```python
from build123d import *

# Parameters (mm, degrees)
SKETCH1_R           = 3.429
BOSS_EXTRUDE1_DEPTH = 50.8
SKETCH2_W           = 50.8
SKETCH2_H           = 43.18
CUT_EXTRUDE1_DEPTH  = 120.811560377
SKETCH3_R           = 2
CUT_EXTRUDE2_DEPTH  = 114.592253257
FILLET1_START       = -1
FILLET1_DEPTH       = 41.6399999
FILLET1_START_2     = 4.794504
FILLET1_2_DEPTH     = 47.205496
FILLET1_START_3     = 40.6399999
FILLET1_3_DEPTH     = 2.5400001
FILLET1_START_4     = -61.640591048
FILLET1_5_DEPTH     = 46.400591048


with BuildPart() as part:
    # Sketch1 → Boss-Extrude1 (new body)
    with BuildSketch(Plane(origin=(0, 0, 0), x_dir=(1, 0, 0), z_dir=(0, 1, 0))):
        Polygon((0, 0), (87.988181024, 0), (87.988181024, 12.7), (0, 63.5), align=None)
        with Locations(Location((40.184090512, 31.500886423, 0), (0, 0, 270))):
            Circle(SKETCH1_R, mode=Mode.SUBTRACT)
    extrude(amount=BOSS_EXTRUDE1_DEPTH)

    # Sketch2 → Cut-Extrude1 (cut, through all)
    with BuildSketch(Plane(origin=(87.988181024, 0, 0), x_dir=(0, 0, -1), z_dir=(1, 0, 0))):
        with Locations((38.1, 21.59)):
            Rectangle(SKETCH2_W, SKETCH2_H)
    extrude(amount=-CUT_EXTRUDE1_DEPTH, mode=Mode.SUBTRACT)

    # Sketch3 → Cut-Extrude2 (cut, through all)
    with BuildSketch(Plane(origin=(0, 0, -12.7), x_dir=(-1, 0, 0), z_dir=(0, 0, -1))):
        with Locations((-69.394090512, 21.59)):
            Circle(SKETCH3_R)
        with Locations((-18.594090512, 21.59)):
            Circle(SKETCH3_R)
    extrude(amount=-CUT_EXTRUDE2_DEPTH, mode=Mode.SUBTRACT)

    # Fillet1: read off the stored shape, not the designer's step
    # Fillet1 outline → Fillet1 (cut)
    with BuildSketch(Plane(origin=(0, 0, 0), x_dir=(1, 0, 0), z_dir=(0, 1, 0)).offset(FILLET1_START)):
        with BuildLine():
            ThreePointArc((85.448181024, 12.7), (87.244232248, 11.956051225), (87.988181024, 10.16))
            Line((87.988181024, 10.16), (87.988181024, 12.7))
            Line((87.988181024, 12.7), (85.448181024, 12.7))
        make_face()
        with BuildLine():
            ThreePointArc((0, 10.16), (0.743948776, 11.956051224), (2.54, 12.7))
            Line((2.54, 12.7), (0, 12.7))
            Line((0, 12.7), (0, 10.16))
        make_face()
        with BuildLine():
            Line((87.988181024, 0), (87.988181024, 2.54))
            ThreePointArc((87.988181024, 2.54), (87.244232248, 0.743948775), (85.448181024, 0))
            Line((85.448181024, 0), (87.988181024, 0))
        make_face()
        with BuildLine():
            ThreePointArc((2.54, 0), (0.743948776, 0.743948776), (0, 2.54))
            Line((0, 2.54), (0, 0))
            Line((0, 0), (2.54, 0))
        make_face()
    extrude(amount=FILLET1_DEPTH, mode=Mode.SUBTRACT)

    # Fillet1 2 outline → Fillet1 2 (cut)
    with BuildSketch(Plane(origin=(0, 0, 0), x_dir=(1, 0, 0), z_dir=(0, 1, 0)).offset(FILLET1_START_2)):
        with BuildLine():
            Line((87.988181024, 11.233530316), (87.988181024, 12.7))
            Line((87.988181024, 12.7), (86.718181024, 13.433234842))
            ThreePointArc((86.718181024, 13.433234842), (87.64788555, 12.503530316), (87.988181024, 11.233530316))
        make_face()
        with BuildLine():
            Line((87.988181024, 0), (87.988181024, 2.54))
            ThreePointArc((87.988181024, 2.54), (87.244232248, 0.743948775), (85.448181024, 0))
            Line((85.448181024, 0), (87.988181024, 0))
        make_face()
        with BuildLine():
            ThreePointArc((2.54, 0), (0.743948776, 0.743948776), (0, 2.54))
            Line((0, 2.54), (0, 0))
            Line((0, 0), (2.54, 0))
        make_face()
        with BuildLine():
            Line((0, 63.5), (0, 59.100590949))
            ThreePointArc((0, 59.100590949), (1.27, 61.300295474), (3.81, 61.300295474))
            Line((3.81, 61.300295474), (0, 63.5))
        make_face()
    extrude(amount=FILLET1_2_DEPTH, mode=Mode.SUBTRACT)

    # Fillet1 3 outline → Fillet1 3 (add)
    with BuildSketch(Plane(origin=(0, 0, 0), x_dir=(1, 0, 0), z_dir=(0, 1, 0)).offset(FILLET1_START_3)):
        with BuildLine():
            Line((0, 12.7), (87.52208234, 12.7))
            ThreePointArc((87.52208234, 12.7), (87.159854864, 13.110168978), (86.718181024, 13.433234842))
            Line((86.718181024, 13.433234842), (3.81, 61.300295474))
            ThreePointArc((3.81, 61.300295474), (1.27, 61.300295474), (0, 59.100590949))
            Line((0, 59.100590949), (0, 12.7))
        make_face()
    extrude(amount=FILLET1_3_DEPTH)

    # Fillet1 4 outline → Fillet1 4 (revolve, cut)
    with BuildSketch(Plane(origin=(0, 40.64, -15.24), x_dir=(0, 1, 0), z_dir=(0, 0, -1))):
        with BuildLine():
            Line((5.08, 87.988181024), (0, 87.988181024))
            Line((0, 87.988181024), (0, 0))
            Line((0, 0), (5.08, 0))
            ThreePointArc((5.08, 0), (3.283948776, 0.743948776), (2.54, 2.54))
            Line((2.54, 2.54), (2.54, 85.448181024))
            ThreePointArc((2.54, 85.448181024), (3.283948775, 87.244232248), (5.08, 87.988181024))
        make_face()
    revolve(axis=Axis((0, 40.64, -15.24), (1, 0, 0)), mode=Mode.SUBTRACT)

    # Fillet1 5 outline → Fillet1 5 (cut)
    with BuildSketch(Plane.XY.offset(FILLET1_START_4)):
        with BuildLine():
            Line((85, 43.18), (2.54, 43.18))
            ThreePointArc((2.54, 43.18), (0.743948776, 43.923948776), (0, 45.72))
            Line((0, 45.72), (0, 40.6399999))
            Line((0, 40.6399999), (85, 40.6399999))
            Line((85, 40.6399999), (85, 43.18))
        make_face()
    extrude(amount=FILLET1_5_DEPTH, mode=Mode.SUBTRACT)


solid = part.part
```
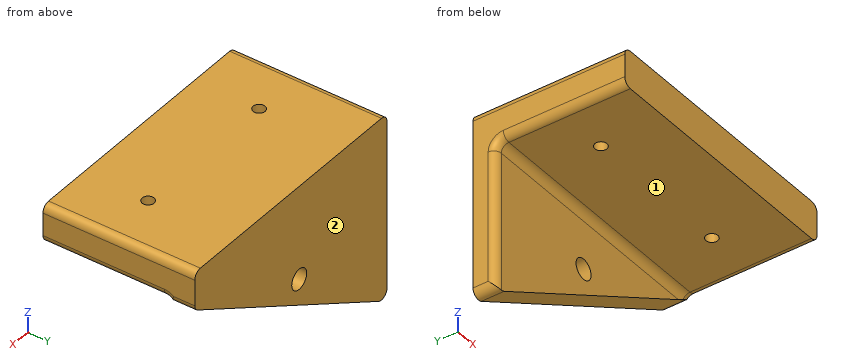
Part model, mm, in its own coordinate system. Face numbers are marked on the shaded views. A direction names the side the tool comes from. Round coordinates to 2 decimals unless told otherwise and drop trailing zeros. Write each loop counter-clockwise with the first axis right and the second up, starting at its lowest first coordinate (ties: lowest second). Pieces come first, ordered by that corner, then holes.
Item 1: Drop flat-ended pins along their axis: pin 1 Ø4.5 at (x, y) = (69.39, 21.59) entering from -Z; pin 2 Ø5 at (x, z) = (38, -40) entering from -Y; pin 3 Ø5 at (x, y) = (46, 41.5) entering from -Z; pin 4 Ø11 at (x, z) = (40.18, -31.5) entering from +Y. Give the stop position or say it passes through.
Results:
pin 1: stops at z = -12.7
pin 2: stops at y = 43.18
pin 3: stops at z = -38.01
pin 4: stops at y = 50.8
Item 2: Cut at C-C, the plane y = 27.5. Give the cut face in (x, z), plus the area to 3 significant figures.
Results:
outline: (0, -10.16) arc R2.54 ccw to (2.54, -12.7) - (85.45, -12.7) arc R2.54 ccw to (87.99, -10.16) - (87.99, -2.54) arc R2.54 ccw to (85.45, 0) - (2.54, 0) arc R2.54 ccw to (0, -2.54) - close
area: 1,110 mm2
Item 3: Which spindle directions (+Z, -Z, +X, -X, +Y, -Y) get a long thin tool onto all of the face, cutting with end or side? Do the marked faces 1 and 2. Say none if no direction does.
Results:
face 1: -Z, +X, -X, -Y
face 2: +Z, -Z, +X, -X, +Y
Item 4: Cut at B-B, the plane x = 23. Give the cut face in (y, z), plus the area to 3 significant figures.
Results:
outline: (0, -12.7) - (40.64, -12.7) arc R2.54 cw to (43.18, -15.24) - (43.18, -50.22) - (50.8, -50.22) - (50.8, 0) - (0, 0) - close
area: 932 mm2
Item 5: Cut at D-D, the plane z = -47.5. Give the cut face in (x, y).
Results:
outline: (0, 45.72) arc R2.54 ccw to (2.54, 43.18) - (27.71, 43.18) - (27.71, 50.8) - (0, 50.8) - close
Item 6: Probe L1, parallel to X at y = 31.5, z = -10.5; L2, parallel to Z at x = 49.5, y = 30.5; L3, parallel to Y at x = 17.5, z = -10.5. List the from-to ranges inside material, lowest first.
Results:
L1: x = 0.02 to 87.97
L2: z = -12.7 to 0
L3: y = 0 to 19.92, 23.26 to 50.8
Item 7: Cut at A-A, the plane y = 21.59. Give the cut face in (x, z).
Results:
outline: (0, -10.16) arc R2.54 ccw to (2.54, -12.7) - (16.59, -12.7) - (16.59, 0) - (2.54, 0) arc R2.54 ccw to (0, -2.54) - close; (20.59, -12.7) - (67.39, -12.7) - (67.39, 0) - (20.59, 0) - close; (71.39, -12.7) - (85.45, -12.7) arc R2.54 ccw to (87.99, -10.16) - (87.99, -2.54) arc R2.54 ccw to (85.45, 0) - (71.39, 0) - close
